Here's the drawing with two shaded views (mm, measured from the low corner). I have some questions. A direction names the side the tool comes from. Round coordinates to 2 decimals unless told otherwise and drop trailing zeros. Order: outer loops, then holes, each group sorted by start corner. A loop starts at its lowest first (then second) coordinate and runs counter-clockwise, first axis right, second up.
Q1. If we section it at D-D (y = 18.5): Please give me the cut outline in (x, z).
Q2. If I drill on line 1 (X direction, y = 22, z = 4.75); line 2 (Z direction, x = 31.5, y = 3.55) (3 decimals); line 3 (X direction, y = 27.5, z = 13), over which ranges is the centre line in solid material (lowest first)?
Q3. If we section it at B-B (z = 6): Please give me the cut outline in (x, y).
Q4. Will these pins go through, and if not, where does the flat tip stop? P1, Ø3, axis at x = 5, z = 5, coming from the +Y side; P2, Ø4.5, axis at y = 11.5, z = 5, coming from the -X side; P3, Ø6, axis at y = 10.5, z = 13, coming from the +X side.
Q5. If we section it at A-A (x = 5): Please give me the cut outline in (y, z) (3 decimals).
Q6. For the marked faces 4, 5 and 6, which set-ups out of +Z, -Z, +X, -X, +Y, -Y let a thin tool reach every point of the face, with its end or its side?
Q7. If we section it at C-C (z = 1.25): Please give me the cut outline in (x, y).
Q8. We'd pull the mould along Z, two halves only. Please class the marked faces 1, 2 and 3: pulls with the +Z half, pulls with the -Z half, needs draft (parallel to the pull), parting line crosses it, or undercut.
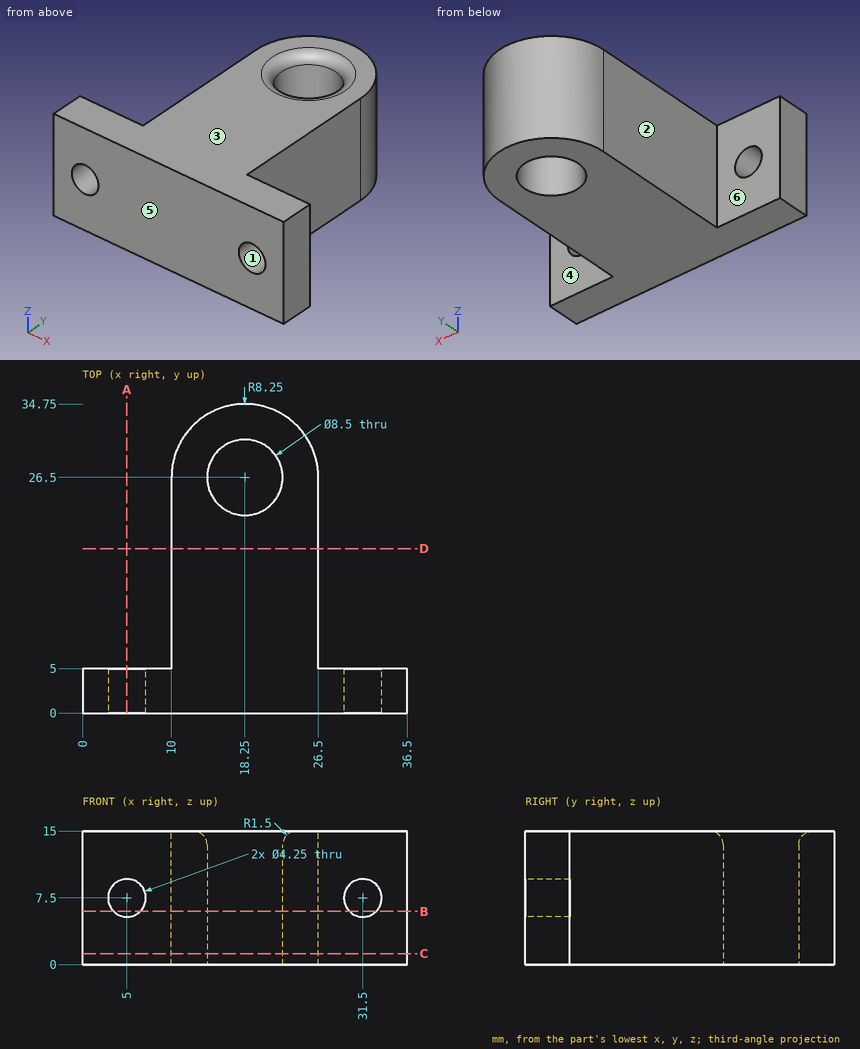
Solution:
1. outline: (10, 0) - (26.5, 0) - (26.5, 15) - (10, 15) - close
2. line 1: x = 10 to 26.5
2. line 2: z = 0 to 5.375, 9.625 to 15
2. line 3: x = 10.06 to 14.12, 22.38 to 26.44
3. outline: (0, 0) - (3.49, 0) - (3.49, 5) - (0, 5) - close; (6.51, 0) - (29.99, 0) - (29.99, 5) - (26.5, 5) - (26.5, 26.5) arc R8.25 ccw to (10, 26.5) - (10, 5) - (6.51, 5) - close; (33.01, 0) - (36.5, 0) - (36.5, 5) - (33.01, 5) - close; hole circle Ø8.5 at (18.25, 26.5)
4. P1: stops at y = 5
4. P2: stops at x = 10
4. P3: stops at x = 26.5
5. outline: (0, 0) - (5, 0) - (5, 5.375) - (0, 5.375) - close; (0, 9.625) - (5, 9.625) - (5, 15) - (0, 15) - close
6. face 4: +Z, -Z, +X, +Y
6. face 5: +Z, -Z, +X, -X, -Y
6. face 6: +Z, -Z, -X, +Y
7. outline: (0, 0) - (36.5, 0) - (36.5, 5) - (26.5, 5) - (26.5, 26.5) arc R8.25 ccw to (10, 26.5) - (10, 5) - (0, 5) - close; hole circle Ø8.5 at (18.25, 26.5)
8. face 1: undercut
8. face 2: needs draft
8. face 3: pulls with the +Z half
